```python
from build123d import *

# Parameters (mm, degrees)
SKETCH1_W           = 71
SKETCH1_H           = 250
BOSS_EXTRUDE1_DEPTH = 5
SKETCH2_W           = 65
SKETCH2_H           = 45
BOSS_EXTRUDE3_DEPTH = 2
LPATTERN1_COUNT     = 5
LPATTERN1_PITCH     = 50
SKETCH3_W           = 69
SKETCH3_H           = 48.754858224
BOSS_EXTRUDE8_DEPTH = 25
LPATTERN5_COUNT     = 5
LPATTERN5_PITCH     = 50


with BuildPart() as part:
    # Sketch1 → Boss-Extrude1 (new body)
    with BuildSketch(Plane(origin=(0, 0, 0), x_dir=(1, 0, 0), z_dir=(0, 1, 0))):
        Rectangle(SKETCH1_W, SKETCH1_H)
    extrude(amount=BOSS_EXTRUDE1_DEPTH)

    # Sketch2 → Boss-Extrude3 (add)
    with BuildSketch(Plane(origin=(0, 5, 0), x_dir=(1, 0, 0), z_dir=(0, 1, 0))):
        with Locations((0, -100)):
            Rectangle(SKETCH2_W, SKETCH2_H)
    boss_extrude3 = extrude(amount=BOSS_EXTRUDE3_DEPTH)

    # LPattern1: Boss-Extrude3 ×5
    with Locations(*[(0, 0, -i * LPATTERN1_PITCH) for i in range(1, LPATTERN1_COUNT)]):
        add(boss_extrude3)

    # Sketch3 → Boss-Extrude8 (add)
    with BuildSketch(Plane(origin=(0, 7, 0), x_dir=(1, 0, 0), z_dir=(0, 1, 0))):
        with Locations((0, -99.635002086)):
            Rectangle(SKETCH3_W, SKETCH3_H)
    boss_extrude8 = extrude(amount=BOSS_EXTRUDE8_DEPTH)

    # LPattern5: Boss-Extrude8 ×5
    with Locations(*[(0, 0, -i * LPATTERN5_PITCH) for i in range(1, LPATTERN5_COUNT)]):
        add(boss_extrude8)


solid = part.part
```
The listing builds one solid part. Answer for the finished solid, in the listing's coordinates (mm). A direction names the side the tool comes from. Coordinates: 2 decimals unless noted, no trailing zeros. Loops run counter-clockwise (first coordinate to the right, second up) from the corner with the lowest first, then second, coordinate; pieces in that order, holes last. Notation, with made-up numbers: (-20.75, -14.75) - (28.25, -14.75) arc R33 ccw to (28.25, 20.25) - close; hole circle Ø8 at (-18, -10.5). An arc over 180 degrees is marked (long way). Use a Markdown table: item, result. Add a question column.
1) The mould has two halves that part along Y. Classify faces 1 (the flat face through (0, 2, -125)), 2 (the flat face through (-3, 7, 123)), 3 (the flat face through (0, 32, 49)): released by +Y, released by -Y, zero draft, split by the parting line, or undercut.
2) Given pin 1 (12 mm diameter, centred on x = -22.5, y = 13.5, fed in from -Z); pin 2 (12.5 mm diameter, centred on y = 18.5, z = 101.5, fed in from -X); pin 3 (4 mm diameter, centred on x = -17, y = 25, fed in from +Z), each flat-ended and moving along its own axis, determine where each tip first touches the part or whether it passes through.
3) For faces 4 (the flat face through (0, 19, 124.012)), 5 (the flat face through (34.5, 19, 100)), 6 (the flat face through (0, 19, 24.012)), 7 (the flat face through (-34.5, 19, -100)), determine the directions among +Z, -Z, +X, -X, +Y, -Y from which every point of the face is accessible in a straight line to the end or side of a thin tool.
4) Find the intervals of material crossed by line 1 (Z direction, x = 3, y = 15); line 2 (Y direction, x = -15, z = -24); line 3 (X direction, y = 10, z = -100.5), in increasing order.
5) The part is cut by section B-B, the plane z = -65. Give the vertices of the cut face in (x, y), and give its area (3 significant figures).
6) The part is cut by section A-A, the plane y = 26.5. Give the vertices of the cut face in (x, z), and give its area (3 significant figures).
Here are the results:
| question | item | result |
|---|---|---|
| 1 | face 1 | zero draft |
| 1 | face 2 | undercut |
| 1 | face 3 | released by +Y |
| 2 | pin 1 | stops at z = -124.74 |
| 2 | pin 2 | stops at x = -34.5 |
| 2 | pin 3 | stops at z = 124.01 |
| 3 | face 4 | +Z, +X, -X, +Y |
| 3 | face 5 | +Z, -Z, +X, +Y |
| 3 | face 6 | +X, -X, +Y |
| 3 | face 7 | +Z, -Z, -X, +Y |
| 4 | line 1 | z = -124.74 to -75.99, -74.74 to -25.99, -24.74 to 24.01, 25.26 to 74.01, 75.26 to 124.01 |
| 4 | line 2 | y = 0 to 5, 7 to 32 |
| 4 | line 3 | x = -34.5 to 34.5 |
| 5 | outline | (-35.5, 0) - (35.5, 0) - (35.5, 5) - (32.5, 5) - (32.5, 7) - (34.5, 7) - (34.5, 32) - (-34.5, 32) - (-34.5, 7) - (-32.5, 7) - (-32.5, 5) - (-35.5, 5) - close |
| 5 | area | 2,210 mm^2 |
| 6 | outline | (-34.5, -124.74) - (34.5, -124.74) - (34.5, -75.99) - (-34.5, -75.99) - close; (-34.5, -74.74) - (34.5, -74.74) - (34.5, -25.99) - (-34.5, -25.99) - close; (-34.5, -24.74) - (34.5, -24.74) - (34.5, 24.01) - (-34.5, 24.01) - close; (-34.5, 25.26) - (34.5, 25.26) - (34.5, 74.01) - (-34.5, 74.01) - close; (-34.5, 75.26) - (34.5, 75.26) - (34.5, 124.01) - (-34.5, 124.01) - close |
| 6 | area | 16,800 mm^2 |
